Source: CAD feature listing. Evaluate the final solid. Frame: model axes, mm. Face numbers are marked on the shaded views. A direction names the side the tool comes from. Round coordinates to 2 decimals unless told otherwise and drop trailing zeros. Write each loop counter-clockwise with the first axis right and the second up, starting at its lowest first coordinate (ties: lowest second). Pieces come first, ordered by that corner, then holes. Notation, with made-up numbers: M 32,14.5 L 55,14.5 A16 cw 55,31.5 Z; hole C -13,-19.75 d9. An arc over 180 degrees is marked long. Use a Markdown table: item, result.
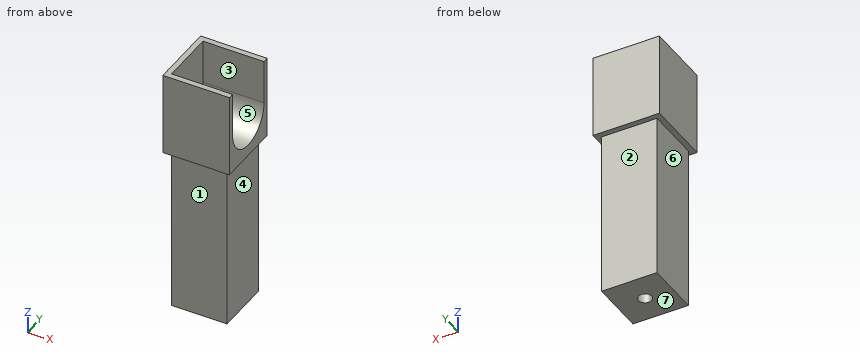
```python
from build123d import *

# Parameters (mm, degrees)
F0_W      = 5
F0_H      = 22.5
F1_DEPTH  = 5
F2_R      = 0.6
F3_DEPTH  = 20
F4_W      = 5
F4_H      = 5
F5_DEPTH  = 5
F6_W      = 5
F6_H      = 5.0048647351
F7_DEPTH  = 0.5
F9_DEPTH  = 0.5
F11_DEPTH = 0.5
F13_DEPTH = 0.5
F15_DEPTH = 25
F16_DEPTH = 4
F17_DEPTH = 7.5
F19_DEPTH = 0.5


with BuildPart() as f1:
    # F0 (on Front) → F1 (new body)
    with BuildSketch(Plane.XZ):
        with Locations((-0.7514320314, 3.0499891839)):
            Rectangle(F0_W, F0_H)
    extrude(amount=F1_DEPTH)

    # F2 (on face) → F3 (cut)
    with BuildSketch(Plane(origin=(0, 0, -8.2000108161), x_dir=(1, 0, 0), z_dir=(0, 0, -1))):
        with Locations((-0.7514320314, 2.5)):
            Circle(F2_R)
    extrude(amount=-F3_DEPTH, mode=Mode.SUBTRACT)

    # F4 (on face) → F5 (join)
    with BuildSketch(Plane.XZ.offset(5)):
        with Locations((-0.7514320314, 16.7999891839)):
            Rectangle(F4_W, F4_H)
    extrude(amount=-F5_DEPTH)

    # F6 (on face) → F7 (join)
    with BuildSketch(Plane.YZ.offset(1.7485679686)):
        with Locations((-2.5, 16.7975568164)):
            Rectangle(F6_W, F6_H)
    extrude(amount=F7_DEPTH)

    # F8 (on face) → F9 (join)
    with BuildSketch(Plane(origin=(0, 0, 0), x_dir=(-1, 0, 0), z_dir=(0, 1, 0))):
        Polygon((-2.2485679686, 14.2951244488), (-1.7485679686, 14.2951244488), (3.2514320314, 14.2951244488), (3.2514320314, 19.2999891839), (-2.2485679686, 19.2999891839), align=None)
    extrude(amount=F9_DEPTH)

    # F10 (on face) → F11 (join)
    with BuildSketch(Plane.XZ.offset(5)):
        Polygon((-3.2514320314, 14.2951244488), (1.7485679686, 14.2951244488), (2.2485679686, 14.2951244488), (2.2485679686, 19.2999891839), (-3.2514320314, 19.2999891839), align=None)
    extrude(amount=F11_DEPTH)

    # F12 (on face) → F13 (join)
    with BuildSketch(Plane(origin=(-3.2514320314, 0, 0), x_dir=(0, -1, 0), z_dir=(-1, 0, 0))):
        Polygon((-0.5, 14.2951244488), (0, 14.2951244488), (5, 14.2951244488), (5.5, 14.2951244488), (5.5, 19.2999891839), (-0.5, 19.2999891839), align=None)
    extrude(amount=F13_DEPTH)

    # F14 (on face) → F15 (cut)
    with BuildSketch(Plane(origin=(-3.7514320314, 0, 0), x_dir=(0, -1, 0), z_dir=(-1, 0, 0))):
        with BuildLine():
            Line((-0.5, 17.7951244488), (0, 17.7951244488))
            ThreePointArc((0, 17.7951244488), (2.5, 15.2951244488), (5, 17.7951244488))
            Line((5, 17.7951244488), (5.5, 17.7951244488))
            Line((5.5, 17.7951244488), (5.5, 19.2999891839))
            Line((5.5, 19.2999891839), (-0.5, 19.2999891839))
            Line((-0.5, 19.2999891839), (-0.5, 17.7951244488))
        make_face()
    extrude(amount=-F15_DEPTH, mode=Mode.SUBTRACT)

    # F16 (add): faces of the model
    f16_faces = [f1.faces().sort_by_distance(p)[0] for p in [
        (-0.7514320314, -5.25, 17.7951244488),
        (-0.7514320314, 0.25, 17.7951244488),
    ]]
    extrude(f16_faces, amount=F16_DEPTH)

    # F17 (cut): a face of the model
    f17_faces = [f1.faces().sort_by_distance(p)[0] for p in [
        (-3.1807213533, -2.5, -8.2000108161),
    ]]
    extrude(f17_faces, amount=-F17_DEPTH, mode=Mode.SUBTRACT)

    # F18 (on face) → F19 (join)
    with BuildSketch(Plane(origin=(-3.7514320314, 0, 0), x_dir=(0, -1, 0), z_dir=(-1, 0, 0))):
        with BuildLine():
            Line((5, 21.7951244488), (0, 21.7951244488))
            Line((0, 21.7951244488), (0, 17.7951244488))
            ThreePointArc((0, 17.7951244488), (2.5, 15.2951244488), (5, 17.7951244488))
            Line((5, 17.7951244488), (5, 21.7951244488))
        make_face()
    extrude(amount=-F19_DEPTH)


solid = f1.part
```
Q1. Line query: L1, parallel to X at y = -2.5, z = 3.5; L2, parallel to Y at x = -3.1, z = 12.5; L3, parallel to X at y = -1.2, z = 4. Output: solid intervals per line, ascending.
Results are:
| item | result |
|---|---|
| L1 | -3.25 to -1.35, -0.15 to 1.75 |
| L2 | -5 to 0 |
| L3 | -3.25 to 1.75 |
Q2. Reachability of the marked faces 5, 6 and 7 from +Z, -Z, +X, -X, +Y, -Y: full face, straight path, thin tool, end or side. Return the list, or none.
Results are:
| item | result |
|---|---|
| face 5 | +Z, +X |
| face 6 | -Z, -X, +Y, -Y |
| face 7 | -Z, +X, -X, +Y, -Y |
Q3. Section A-A on y = -2.5. Return loops of the section in (x, z), plus the area to 3 significant figures.
Results are:
| item | result |
|---|---|
| outline | M -3.75,14.3 L -3.25,14.3 L -3.25,-0.7 L -1.35,-0.7 L -1.35,11.8 L -0.15,11.8 L -0.15,-0.7 L 1.75,-0.7 L 1.75,14.3 L 2.25,14.3 L 2.25,15.3 L -3.25,15.3 L -3.25,21.8 L -3.75,21.8 Z |
| area | 69.2 mm^2 |
Q4. Section C-C on z = 3.25. Return loops of the section in (x, y), plus the area to 3 significant figures.
Results are:
| item | result |
|---|---|
| outline | M -3.25,-5 L 1.75,-5 L 1.75,0 L -3.25,0 Z; hole C -0.75,-2.5 d1.2 |
| area | 23.9 mm^2 |
Q5. Mould query, pull axis Y, two halves, no side actions, for the marked faces 1, 2, 3 and 4. Classes: +Y half, -Y half, draft (parallel to the pull), parting line (faces both ways), or undercut.
Results are:
| item | result |
|---|---|
| face 1 | -Y half |
| face 2 | +Y half |
| face 3 | undercut |
| face 4 | draft |
Q6. Section B-B on x = -2.7. Return loops of the section in (y, z), plus the area to 3 significant figures.
Results are:
| item | result |
|---|---|
| outline | M -5.5,14.3 L -5,14.3 L -5,-0.7 L 0,-0.7 L 0,14.3 L 0.5,14.3 L 0.5,21.8 L 0,21.8 L 0,17.8 A2.5 cw -5,17.8 L -5,21.8 L -5.5,21.8 Z |
| area | 90.2 mm^2 |
Q7. Section D-D on z = 16.5. Return loops of the section in (x, y), plus the area to 3 significant figures.
Results are:
| item | result |
|---|---|
| outline | M -3.75,-5.5 L 2.25,-5.5 L 2.25,-4.64 L -3.25,-4.64 L -3.25,-0.36 L 2.25,-0.36 L 2.25,0.5 L -3.75,0.5 Z |
| area | 12.5 mm^2 |
Q8. First-contact query: pin 1 Ø3 at (x, z) = (-3, 8) entering from +Y; pin 2 Ø1.5 at (x, z) = (-3, 12) entering from -Y; pin 3 Ø1.5 at (y, z) = (-3, 19) entering from +X. Flat tips, straight axial feed; report the tip coordinate or a pass-through.
Results are:
| item | result |
|---|---|
| pin 1 | y = 0 |
| pin 2 | y = -5 |
| pin 3 | x = -3.25 |
